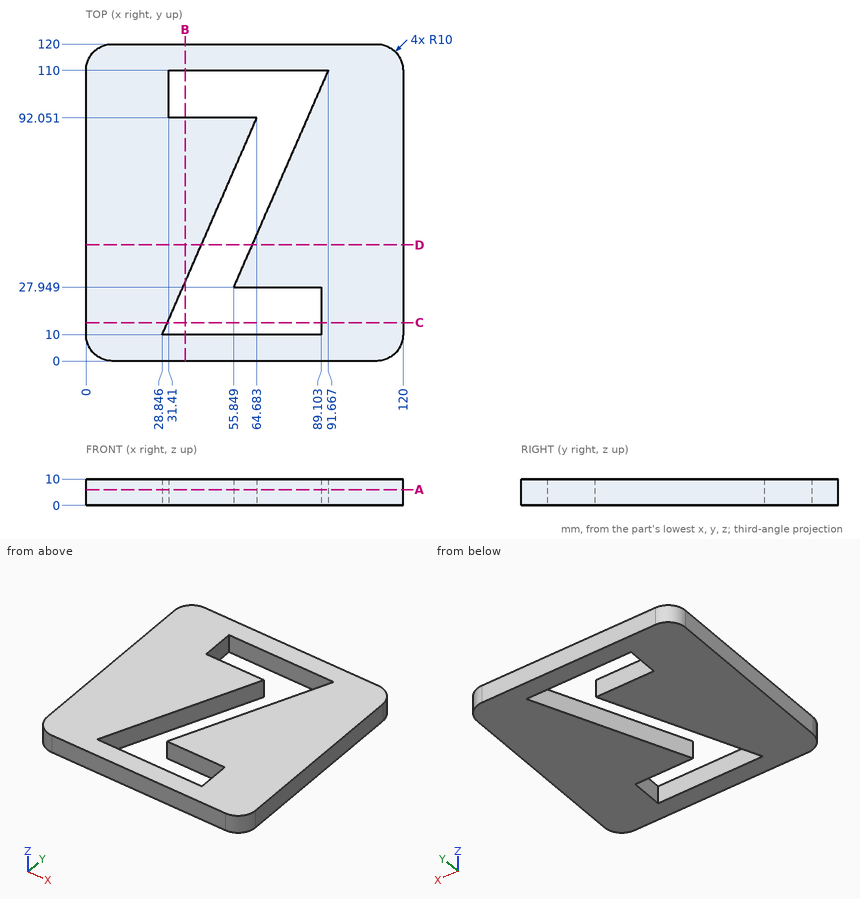
Could you check a few things on this drawing? It's one solid part, dimensions in mm from its lowest x, y, z. Round coordinates to 2 decimals unless told otherwise and drop trailing zeros. Write each loop counter-clockwise with the first axis right and the second up, starting at its lowest first coordinate (ties: lowest second). Pieces come first, ordered by that corner, then holes.
Q1. If we section it at D-D on y = 44: Write out the boundary of the cut face in (x, z).
Q2. Please list where these lines run through material, in increasing order: probe 1 along X at (y, z) = (76, 5) (1 decimal); probe 2 along X at (y, z) = (53, 3.75) (1 decimal); probe 3 along Y at (x, z) = (111.5, 1.25).
Q3. If we section it at B-B on x = 37.5: Write out the boundary of the cut face in (y, z).
Q4. If we section it at C-C on y = 14.5: Write out the boundary of the cut face in (x, z).
Q5. If we section it at A-A on z = 6: Write out the boundary of the cut face in (x, y), plus the area to 3 significant figures.
Answer below:
1. outline: (0, 0) - (43.7, 0) - (43.7, 10) - (0, 10) - close; (62.86, 0) - (120, 0) - (120, 10) - (62.86, 10) - close
2. probe 1: x = 0 to 57.7, 76.8 to 120
2. probe 2: x = 0 to 47.6, 66.8 to 120
2. probe 3: y = 0.11 to 119.89
3. outline: (0, 0) - (10, 0) - (10, 10) - (0, 10) - close; (29.81, 0) - (92.05, 0) - (92.05, 10) - (29.81, 10) - close; (110, 0) - (120, 0) - (120, 10) - (110, 10) - close
4. outline: (0, 0) - (30.81, 0) - (30.81, 10) - (0, 10) - close; (89.1, 0) - (120, 0) - (120, 10) - (89.1, 10) - close
5. outline: (0, 10) arc R10 ccw to (10, 0) - (110, 0) arc R10 ccw to (120, 10) - (120, 110) arc R10 ccw to (110, 120) - (10, 120) arc R10 ccw to (0, 110) - close; hole (28.85, 10) - (89.1, 10) - (89.1, 27.95) - (55.85, 27.95) - (91.67, 110) - (31.41, 110) - (31.41, 92.05) - (64.68, 92.05) - close
5. area: 11,100 mm2
